The listing builds one solid part. Answer for the finished solid, in the listing's coordinates (mm). A direction names the side the tool comes from. Give positions to 0.01 mm unless a question says otherwise; leave off trailing zeros. Write each loop counter-clockwise with the first axis right and the second up, starting at its lowest first coordinate (ties: lowest second). Pieces come first, ordered by that corner, then holes. Notation, with made-up numbers: (32, -30) -> (58, -30) arc R17 ccw to (58, -25) -> close; hole circle Ø9 at (-19, 49.25). An arc over 180 degrees is marked (long way). Put each result on its own line as item: value. Start each with the question number.
1) Find the intervals of material crossed by line 1 along Y through (x, z) = (-36, 3.2); line 2 along X through (y, z) = (2.5, 3.1); line 3 along X through (y, z) = (-0.5, 0.9), in increasing order. Write a range as from..to.
2) A cutting plane is placed at B-B (y = -15.5). Write down the section's boundary in (x, z).
3) Flat-ended cylindrical pins translate along their axes: pin 1 Ø5.5 at (x, y) = (5, -46) entering from -Z; pin 2 Ø6.5 at (x, y) = (0, 0) entering from -Z; pin 3 Ø1.5 at (x, z) = (0, 3.5) entering from +Y; pin 4 Ø1.1 at (x, z) = (-1, 3.5) entering from +Y. Find the tip coordinate at first contact, or state that the pin passes through.
4) For a pull along Y with two mould halves and no side action, classify faces 3 (the cylindrical face through (-33.183, -1.168, 2.028)), 4 (the cylindrical face through (-0.661, -38.977, 2.028)), 5 (the flat face through (10, -33, 2)), 6 (the cylindrical face through (-49.43, -9.4, 1.97)) as released by +Y, released by -Y, zero draft, split by the parting line, or undercut.
5) A cutting plane is placed at A-A (x = -46). Write down the section's boundary in (y, z).
6) A cutting plane is placed at D-D (x = -13). Write down the section's boundary in (y, z).
7) For faces 1 (the flat face through (-33, -10, 2)), 2 (the flat face through (-50, 0, 2)), determine the directions among +Z, -Z, +X, -X, +Y, -Y from which every point of the face is accessible in a straight line to the end or side of a thin tool.
from build123d import *

# Parameters (mm, degrees)
EXTRUDE_1_DEPTH         = 3
SKETCH_2_R              = 2.05
CUT_EXTRUDE_1_DEPTH     = 10
CUT_EXTRUDE_2_DEPTH     = 10
SKETCH_4_R              = 4.1
CUT_EXTRUDE_3_DEPTH     = 10
SKETCH_5_W              = 14
SKETCH_5_H              = 10
SKETCH_5_W_2            = 10
SKETCH_5_H_2            = 14
CUT_EXTRUDE_4_DEPTH     = 10
FILLET_1_R              = 2
FILLET_2_R              = 2
MOVE_START              = 3
MOVE_FACE_1_OUTLINE_R   = 2.05
MOVE_FACE_1_OUTLINE_R_2 = 4.1
MOVE_FACE_1_DEPTH       = 1
SKETCH_9_W              = 14
SKETCH_9_H              = 10
SKETCH_9_W_2            = 10
SKETCH_9_H_2            = 14
EXTRUDE_2_DEPTH         = 4
SKETCH_10_R             = 3.05
CUT_EXTRUDE_6_DEPTH     = 10


# Read off the part's stored shape, not the designer's step: 移动面1
with BuildPart() as part:
    # 草图1 → 凸台-拉伸1 (new body)
    with BuildSketch(Plane.XY):
        Polygon((-50, 10), (10, 10), (10, -50), (-10, -50), (-10, -10), (-50, -10), align=None)
    extrude(amount=EXTRUDE_1_DEPTH)

    # 草图2 → 切除-拉伸1 (cut)
    with BuildSketch(Plane.XY.offset(3)):
        with Locations((-26, -5)):
            Circle(SKETCH_2_R)
        with Locations((-46, 5)):
            Circle(SKETCH_2_R)
        with Locations((-46, -5)):
            Circle(SKETCH_2_R)
        with Locations((-26, 5)):
            Circle(SKETCH_2_R)
        with Locations((5, -26)):
            Circle(SKETCH_2_R)
        with Locations((-5, -46)):
            Circle(SKETCH_2_R)
        with Locations((5, -46)):
            Circle(SKETCH_2_R)
        with Locations((-5, -26)):
            Circle(SKETCH_2_R)
    extrude(amount=-CUT_EXTRUDE_1_DEPTH, mode=Mode.SUBTRACT)

    # 草图3 → 切除-拉伸2 (cut)
    with BuildSketch(Plane.XY.offset(3)):
        with BuildLine():
            Line((-18, 10), (1.259110699, 5.866399258))
            ThreePointArc((1.259110699, 5.866399258), (4.242640687, 4.242640687), (5.866399258, 1.259110699))
            Line((5.866399258, 1.259110699), (10, -18))
            Line((10, -18), (10, 10))
            Line((10, 10), (-18, 10))
        make_face()
        Polygon((-18, -10), (-7.813706378, -7.813706378), (-10, -18), align=None)
    extrude(amount=-CUT_EXTRUDE_2_DEPTH, mode=Mode.SUBTRACT)

    # 草图4 → 切除-拉伸3 (cut)
    with BuildSketch(Plane.XY.offset(3)):
        Circle(SKETCH_4_R)
    extrude(amount=-CUT_EXTRUDE_3_DEPTH, mode=Mode.SUBTRACT)

    # 草图5 → 切除-拉伸4 (cut)
    with BuildSketch(Plane.XY.offset(3)):
        with Locations((-36, 0)):
            Rectangle(SKETCH_5_W, SKETCH_5_H)
        with BuildLine():
            Line((-22, 5.74465424), (-22, -6.767428132))
            Line((-22, -6.767428132), (-5.111190695, -3.14256737))
            ThreePointArc((-5.111190695, -3.14256737), (-5.977725364, -0.516526349), (-5.574495891, 2.219233101))
            Line((-5.574495891, 2.219233101), (-22, 5.74465424))
        make_face()
        with BuildLine():
            Line((2.219233101, -5.574495891), (5.74465424, -22))
            Line((5.74465424, -22), (-6.767428132, -22))
            Line((-6.767428132, -22), (-3.14256737, -5.111190695))
            ThreePointArc((-3.14256737, -5.111190695), (-0.516526349, -5.977725364), (2.219233101, -5.574495891))
        make_face()
        with Locations((0, -36)):
            Rectangle(SKETCH_5_W_2, SKETCH_5_H_2)
    extrude(amount=-CUT_EXTRUDE_4_DEPTH, mode=Mode.SUBTRACT)

    # 圆角1
    fillet_1_edges = [part.edges().sort_by_distance(p)[0] for p in [
        (-29, 5, 1.5),
        (-29, -5, 1.5),
        (-43, -5, 1.5),
        (-43, 5, 1.5),
        (-3.14256737, -5.111190695, 1.5),
        (2.219233101, -5.574495891, 1.5),
        (5.74465424, -22, 1.5),
        (-6.767428132, -22, 1.5),
        (5, -43, 1.5),
        (-5, -43, 1.5),
        (-5, -29, 1.5),
        (5, -29, 1.5),
        (-22, 5.74465424, 1.5),
        (-5.574495891, 2.219233101, 1.5),
        (-5.111190695, -3.14256737, 1.5),
        (-22, -6.767428132, 1.5),
    ]]
    fillet(fillet_1_edges, radius=FILLET_1_R)

    # 圆角2
    fillet_2_edges = [part.edges().sort_by_distance(p)[0] for p in [
        (-50, 10, 1.5),
        (10, -50, 1.5),
        (-10, -50, 1.5),
        (-50, -10, 1.5),
        (-18, -10, 1.5),
        (-7.813706378, -7.813706378, 1.5),
        (-10, -18, 1.5),
        (-18, 10, 1.5),
        (10, -18, 1.5),
    ]]
    fillet(fillet_2_edges, radius=FILLET_2_R)

    # Move Face 1 outline → Move Face 1 (add)
    with BuildSketch(Plane.XY.offset(MOVE_START)):
        with BuildLine():
            Line((-50, 8), (-50, -8))
            ThreePointArc((-50, -8), (-49.414213562, -9.414213562), (-48, -10))
            Line((-48, -10), (-18.21221445, -10))
            ThreePointArc((-18.21221445, -10), (-18.00118464, -9.988835443), (-17.792510884, -9.955466419))
            Line((-17.792510884, -9.955466419), (-10.837978737, -8.462808752))
            ThreePointArc((-10.837978737, -8.462808752), (-9.004061609, -9.004061609), (-8.462808752, -10.837978737))
            Line((-8.462808752, -10.837978737), (-9.955466419, -17.792510884))
            ThreePointArc((-9.955466419, -17.792510884), (-9.988835443, -18.00118464), (-10, -18.21221445))
            Line((-10, -18.21221445), (-10, -48))
            ThreePointArc((-10, -48), (-9.414213562, -49.414213562), (-8, -50))
            Line((-8, -50), (8, -50))
            ThreePointArc((8, -50), (9.414213562, -49.414213562), (10, -48))
            Line((10, -48), (10, -18.21221445))
            ThreePointArc((10, -18.21221445), (9.988835443, -18.00118464), (9.955466419, -17.792510884))
            Line((9.955466419, -17.792510884), (5.866399258, 1.259110699))
            ThreePointArc((5.866399258, 1.259110699), (4.242640687, 4.242640687), (1.259110699, 5.866399258))
            Line((1.259110699, 5.866399258), (-17.792510884, 9.955466419))
            ThreePointArc((-17.792510884, 9.955466419), (-18.00118464, 9.988835443), (-18.21221445, 10))
            Line((-18.21221445, 10), (-48, 10))
            ThreePointArc((-48, 10), (-49.414213562, 9.414213562), (-50, 8))
        make_face()
        with Locations((-5, -46)):
            Circle(MOVE_FACE_1_OUTLINE_R, mode=Mode.SUBTRACT)
        with Locations((5, -46)):
            Circle(MOVE_FACE_1_OUTLINE_R, mode=Mode.SUBTRACT)
        with BuildLine():
            Line((3, -43), (-3, -43))
            ThreePointArc((-3, -43), (-4.414213562, -42.414213562), (-5, -41))
            Line((-5, -41), (-5, -31))
            ThreePointArc((-5, -31), (-4.414213562, -29.585786438), (-3, -29))
            Line((-3, -29), (3, -29))
            ThreePointArc((3, -29), (4.414213562, -29.585786438), (5, -31))
            Line((5, -31), (5, -41))
            ThreePointArc((5, -41), (4.414213562, -42.414213562), (3, -43))
        make_face(mode=Mode.SUBTRACT)
        with Locations((-5, -26)):
            Circle(MOVE_FACE_1_OUTLINE_R, mode=Mode.SUBTRACT)
        with Locations((5, -26)):
            Circle(MOVE_FACE_1_OUTLINE_R, mode=Mode.SUBTRACT)
        with Locations((-46, -5)):
            Circle(MOVE_FACE_1_OUTLINE_R, mode=Mode.SUBTRACT)
        with BuildLine():
            Line((-29, 3), (-29, -3))
            ThreePointArc((-29, -3), (-29.585786438, -4.414213562), (-31, -5))
            Line((-31, -5), (-41, -5))
            ThreePointArc((-41, -5), (-42.414213562, -4.414213562), (-43, -3))
            Line((-43, -3), (-43, 3))
            ThreePointArc((-43, 3), (-42.414213562, 4.414213562), (-41, 5))
            Line((-41, 5), (-31, 5))
            ThreePointArc((-31, 5), (-29.585786438, 4.414213562), (-29, 3))
        make_face(mode=Mode.SUBTRACT)
        with Locations((-46, 5)):
            Circle(MOVE_FACE_1_OUTLINE_R, mode=Mode.SUBTRACT)
        with Locations((-26, -5)):
            Circle(MOVE_FACE_1_OUTLINE_R, mode=Mode.SUBTRACT)
        with Locations((-26, 5)):
            Circle(MOVE_FACE_1_OUTLINE_R, mode=Mode.SUBTRACT)
        with BuildLine():
            ThreePointArc((-3.634280684, -7.40216211), (-2.764762592, -6.142366874), (-1.259110699, -5.866399258))
            ThreePointArc((-1.259110699, -5.866399258), (-0.375737475, -5.988223555), (0.515935261, -5.97777641))
            ThreePointArc((0.515935261, -5.97777641), (1.87690568, -6.362171411), (2.6433801, -7.55066498))
            Line((2.6433801, -7.55066498), (5.225311026, -19.580296434))
            ThreePointArc((5.225311026, -19.580296434), (4.825384245, -21.257098418), (3.269844607, -22))
            Line((3.269844607, -22), (-4.292618499, -22))
            ThreePointArc((-4.292618499, -22), (-5.848158137, -21.257098418), (-6.248084918, -19.580296434))
            Line((-6.248084918, -19.580296434), (-3.634280684, -7.40216211))
        make_face(mode=Mode.SUBTRACT)
        with BuildLine():
            ThreePointArc((-7.55066498, 2.6433801), (-6.362171411, 1.87690568), (-5.97777641, 0.515935261))
            ThreePointArc((-5.97777641, 0.515935261), (-5.988223555, -0.375737475), (-5.866399258, -1.259110699))
            ThreePointArc((-5.866399258, -1.259110699), (-6.142366874, -2.764762592), (-7.40216211, -3.634280684))
            Line((-7.40216211, -3.634280684), (-19.580296434, -6.248084918))
            ThreePointArc((-19.580296434, -6.248084918), (-21.257098418, -5.848158137), (-22, -4.292618499))
            Line((-22, -4.292618499), (-22, 3.269844607))
            ThreePointArc((-22, 3.269844607), (-21.257098418, 4.825384245), (-19.580296434, 5.225311026))
            Line((-19.580296434, 5.225311026), (-7.55066498, 2.6433801))
        make_face(mode=Mode.SUBTRACT)
        Circle(MOVE_FACE_1_OUTLINE_R_2, mode=Mode.SUBTRACT)
    extrude(amount=MOVE_FACE_1_DEPTH)

    # 草图9 → 凸台-拉伸2 (add)
    with BuildSketch(Plane.XY.offset(4)):
        with Locations((-36, 0)):
            Rectangle(SKETCH_9_W, SKETCH_9_H)
        with Locations((0, -36)):
            Rectangle(SKETCH_9_W_2, SKETCH_9_H_2)
    extrude(amount=-EXTRUDE_2_DEPTH)

    # 草图10 → 切除-拉伸6 (cut)
    with BuildSketch(Plane.XY.offset(4)):
        with Locations((-36, 0)):
            Circle(SKETCH_10_R)
        with Locations((0, -36)):
            Circle(SKETCH_10_R)
    extrude(amount=-CUT_EXTRUDE_6_DEPTH, mode=Mode.SUBTRACT)


solid = part.part
Reply:
1. line 1: y = -10..-3.05, 3.05..10
1. line 2: x = -50..-37.75, -34.25..-22, -7.12..-3.25, 3.25..5.45
1. line 3: x = -50..-39.01, -32.99..-22, -5.98..-4.07, 4.07..6.24
2. outline: (-9.46, 0) -> (-5.37, 0) -> (-5.37, 4) -> (-9.46, 4) -> close; (4.35, 0) -> (9.46, 0) -> (9.46, 4) -> (4.35, 4) -> close
3. pin 1: stops at z = 0
3. pin 2: passes through
3. pin 3: stops at y = 6.3
3. pin 4: stops at y = 6.47
4. face 3: undercut
4. face 4: undercut
4. face 5: zero draft
4. face 6: released by -Y
5. outline: (-10, 0) -> (-7.05, 0) -> (-7.05, 4) -> (-10, 4) -> close; (-2.95, 0) -> (2.95, 0) -> (2.95, 4) -> (-2.95, 4) -> close; (7.05, 0) -> (10, 0) -> (10, 4) -> (7.05, 4) -> close
6. outline: (-8.93, 0) -> (-4.84, 0) -> (-4.84, 4) -> (-8.93, 4) -> close; (3.81, 0) -> (8.93, 0) -> (8.93, 4) -> (3.81, 4) -> close
7. face 1: +Z, -Z, -X, -Y
7. face 2: +Z, -Z, -X, +Y, -Y
